Verification items for the finished model (mm, model axes). A direction names the side the tool comes from. Coordinates: 2 decimals unless noted, no trailing zeros. Loops run counter-clockwise (first coordinate to the right, second up) from the corner with the lowest first, then second, coordinate; pieces in that order, holes last. Notation, with made-up numbers: (69, 75) - (106, 75) arc R25 ccw to (106, 99) - close; hole circle Ø6 at (79.25, 89). An arc over 180 degrees is marked (long way). One line per item, written item: value. Start each with the question number.
(1) Section check D-D (y = 3.5). Record the boundary of the cut face in (x, z) (3 decimals).
(2) Set-up check for faces 4 (the face through (0, -10.795, 5)), 5 (the face through (15.875, 0, -13)), 6 (the face through (-15.875, 0, -13)), 7 (the face through (0, -6.985, -13)), 8 (the face through (0, 6.985, -13)): record each of +Z, -Z, +X, -X, +Y, -Y from which the full face is reachable in a straight line by a thin tool's end or side.
(3) Draft check along Y on faces 1 (the face through (-22.984, 0.237, 4.747)), 2 (the face through (0, -8, 0)), 3 (the face through (-25.397, 0.279, 3.131)). Enter one of: +Y half, -Y half, draft (parallel to the pull), parting line (faces both ways), or undercut.
(4) Section check B-B (z = 4). Record the boundary of the cut face in (x, y) (3 decimals).
(5) Section check C-C (x = -20). Record the boundary of the cut face in (y, z).
(6) Section check A-A (y = 0). Record the boundary of the cut face in (x, z) (3 decimals), plus the area to 3 significant figures.
(7) Thickness scan on probe 1 along Y at (x, z) = (1, -10) (3 decimals); probe 2 along Z at (x, y) = (-12, 9.25); probe 3 along Z at (x, y) = (9.5, -0.5). Record the ranges inside material, lowest first. Write a range as [from, to].
(8) Gauge pin test, flat ends, axial feed: P1, Ø6, axis at y = 0.5, z = -18, coming from the -X side (3 decimals); P2, Ø1.5, axis at x = 15.5, y = -5, coming from the +Z side; P3, Ø7, axis at y = -2.5, z = -14.5, coming from the +X side (3 decimals). Record the tip position at first contact, or that the pin passes through.
```python
from build123d import *

# Parameters (mm, degrees)
F1_DEPTH = 6.35
F2_W     = 31.75
F2_H     = 13.97
F3_DEPTH = 25.4
F5_DEPTH = 3.2512


# Not quite as in the source:
# - a feature names something its author has since deleted; it is built from what else it names


with BuildPart() as f1:
    # F0 (on Top) → F1 (new body)
    with BuildSketch(Plane.XY):
        with BuildLine():
            Line((-12.7, -12.7), (12.7, -12.7))
            ThreePointArc((12.7, -12.7), (25.4, 0), (12.7, 12.7))
            Line((12.7, 12.7), (-12.7, 12.7))
            ThreePointArc((-12.7, 12.7), (-25.4, 0), (-12.7, -12.7))
        make_face()
    extrude(amount=F1_DEPTH)

    # F2 (on face) → F3 (join)
    with BuildSketch(Plane(origin=(0, 0, 0), x_dir=(1, 0, 0), z_dir=(0, 0, -1))):
        Rectangle(F2_W, F2_H)
    extrude(amount=F3_DEPTH)

    # F4 (on face) → F5 (cut)
    with BuildSketch(Plane.XY.offset(6.35)):
        with BuildLine():
            Line((-12.192, -10.795), (12.192, -10.795))
            ThreePointArc((12.192, -10.795), (22.987, 0), (12.192, 10.795))
            Line((12.192, 10.795), (-12.192, 10.795))
            ThreePointArc((-12.192, 10.795), (-22.987, 0), (-12.192, -10.795))
        make_face()
    extrude(amount=-F5_DEPTH, mode=Mode.SUBTRACT)


solid = f1.part
```
Responses:
1. outline: (-24.908, 0) - (-15.875, 0) - (-15.875, -25.4) - (15.875, -25.4) - (15.875, 0) - (24.908, 0) - (24.908, 6.35) - (22.404, 6.35) - (22.404, 3.099) - (-22.404, 3.099) - (-22.404, 6.35) - (-24.908, 6.35) - close
2. face 4: +Z
2. face 5: -Z, +X, +Y, -Y
2. face 6: -Z, -X, +Y, -Y
2. face 7: -Z, +X, -X, -Y
2. face 8: -Z, +X, -X, +Y
3. face 1: undercut
3. face 2: draft
3. face 3: parting line
4. outline: (-12.7, -12.7) - (12.7, -12.7) arc R12.7 ccw to (12.7, 12.7) - (-12.7, 12.7) arc R12.7 ccw to start; hole (-12.192, -10.795) - (12.192, -10.795) arc R10.795 ccw to (12.192, 10.795) - (-12.192, 10.795) arc R10.795 ccw to start
5. outline: (-10.39, 0) - (10.39, 0) - (10.39, 6.35) - (7.45, 6.35) - (7.45, 3.1) - (-7.45, 3.1) - (-7.45, 6.35) - (-10.39, 6.35) - close
6. outline: (-25.4, 0) - (-15.875, 0) - (-15.875, -25.4) - (15.875, -25.4) - (15.875, 0) - (25.4, 0) - (25.4, 6.35) - (22.987, 6.35) - (22.987, 3.099) - (-22.987, 3.099) - (-22.987, 6.35) - (-25.4, 6.35) - close
6. area: 980 mm²
7. probe 1: y = [-6.985, 6.985]
7. probe 2: z = [0, 3.1]
7. probe 3: z = [-25.4, 3.1]
8. P1: stops at x = -15.875
8. P2: stops at z = 3.1
8. P3: stops at x = 15.875
